Verification items for the finished model (mm, model axes). A direction names the side the tool comes from. Coordinates: 2 decimals unless noted, no trailing zeros. Write each loop counter-clockwise with the first axis right and the second up, starting at its lowest first coordinate (ties: lowest second). Pieces come first, ordered by that corner, then holes. Notation, with made-up numbers: M -19,75.5 L 30,75.5 A17 ccw 30,81.5 Z; hole C -21.5,43.25 d5. An arc over 180 degrees is marked long. Answer in a Markdown table with one row per item.
from build123d import *

# Parameters (mm, degrees)
SKETCH1_W           = 30
SKETCH1_H           = 25
BOSS_EXTRUDE1_DEPTH = 20
SKETCH2_W           = 20
SKETCH2_H           = 25
CUT_EXTRUDE1_DEPTH  = 10
CUT_EXTRUDE2_DEPTH  = 20
CUT_EXTRUDE3_DEPTH  = 40
SKETCH5_W           = 20
SKETCH5_H           = 10
CUT_EXTRUDE4_DEPTH  = 20
BOSS_EXTRUDE2_DEPTH = 10


with BuildPart() as part:
    # Sketch1 → Boss-Extrude1 (new body)
    with BuildSketch(Plane.XY):
        with Locations((15, 12.5)):
            Rectangle(SKETCH1_W, SKETCH1_H)
    extrude(amount=BOSS_EXTRUDE1_DEPTH)

    # Sketch2 → Cut-Extrude1 (cut)
    with BuildSketch(Plane.XY.offset(20)):
        with Locations((10, 12.5)):
            Rectangle(SKETCH2_W, SKETCH2_H)
    extrude(amount=-CUT_EXTRUDE1_DEPTH, mode=Mode.SUBTRACT)

    # Sketch3 → Cut-Extrude2 (cut)
    with BuildSketch(Plane.ZY.offset(-20)):
        Polygon((15, 25), (20, 15), (20, 25), align=None)
    extrude(amount=-CUT_EXTRUDE2_DEPTH, mode=Mode.SUBTRACT)

    # Sketch4 → Cut-Extrude3 (cut)
    with BuildSketch(Plane(origin=(0, 25, 0), x_dir=(1, 0, 0), z_dir=(0, 1, 0))):
        Polygon((0, -10), (10, -10), (0, 0), align=None)
    extrude(amount=-CUT_EXTRUDE3_DEPTH, mode=Mode.SUBTRACT)

    # Sketch5 → Cut-Extrude4 (cut)
    with BuildSketch(Plane.ZY.offset(-20)):
        with Locations((0, 20)):
            Rectangle(SKETCH5_W, SKETCH5_H)
    extrude(amount=CUT_EXTRUDE4_DEPTH, mode=Mode.SUBTRACT)

    # Sketch6 → Boss-Extrude2 (add)
    with BuildSketch(Plane(origin=(0, 15, 0), x_dir=(1, 0, 0), z_dir=(0, 1, 0))):
        Polygon((0, -10), (20, -10), (20, 0), (10, 0), align=None)
    extrude(amount=BOSS_EXTRUDE2_DEPTH)


solid = part.part
1) Thickness scan on L1, parallel to Z at x = 17.75, y = 22; L2, parallel to X at y = 9.25, z = 11.5; L3, parallel to Y at x = 4.5, z = 3. Record the ranges inside material, lowest first. Write a range as [from, to].
Response values:
| item | result |
|---|---|
| L1 | z = [0, 10] |
| L2 | x = [20, 30] |
| L3 | y = [0, 15] |
2) Sectioned sample at A-A (x = 3.75). Record the cut outline in (y, z).
Response values:
| item | result |
|---|---|
| outline | M 0,0 L 15,0 L 15,3.75 L 0,3.75 Z; M 15,6.25 L 25,6.25 L 25,10 L 15,10 Z |
3) Tool access check on faces 1 (the face through (12, 15, 10)), 2 (the face through (5, 20, 5)), 3 (the face through (30, 12, 10)), 4 (the face through (5, 8, 5)). Record the directions out of +Z, -Z, +X, -X, +Y, -Y that give a thin tool (end or side, any length) a straight path to the whole face; none if there is none.
Response values:
| item | result |
|---|---|
| face 1 | +Z, -X, +Y, -Y |
| face 2 | -Z, -X, +Y |
| face 3 | +Z, -Z, +X, +Y, -Y |
| face 4 | +Z, -X, -Y |
4) Sectioned sample at B-B (z = 1.75). Record the cut outline in (x, y), then the cut area to 3 significant figures.
Response values:
| item | result |
|---|---|
| outline | M 1.75,0 L 30,0 L 30,25 L 8.25,25 L 8.25,15 L 1.75,15 Z |
| area | 641 mm² |
5) Depth check by flat-ended pin: pin 1 (2 mm diameter, centred on y = 19, z = 3, fed in from -X); pin 2 (1.5 mm diameter, centred on x = 3.5, z = 2, fed in from +Y); pin 3 (8 mm diameter, centred on y = 9.5, z = 16.5, fed in from -X). Enter the tip coordinate at first touch or a pass-through.
Response values:
| item | result |
|---|---|
| pin 1 | stops at x = 6 |
| pin 2 | stops at y = 15 |
| pin 3 | stops at x = 20 |
6) Sectioned sample at C-C (y = 17.5). Record the cut outline in (x, z).
Response values:
| item | result |
|---|---|
| outline | M 0,10 L 10,0 L 30,0 L 30,18.75 L 20,18.75 L 20,10 Z |
7) Sectioned sample at D-D (x = 24). Record the cut outline in (y, z), then the cut area to 3 significant figures.
Response values:
| item | result |
|---|---|
| outline | M 0,0 L 25,0 L 25,15 L 15,20 L 0,20 Z |
| area | 475 mm² |
